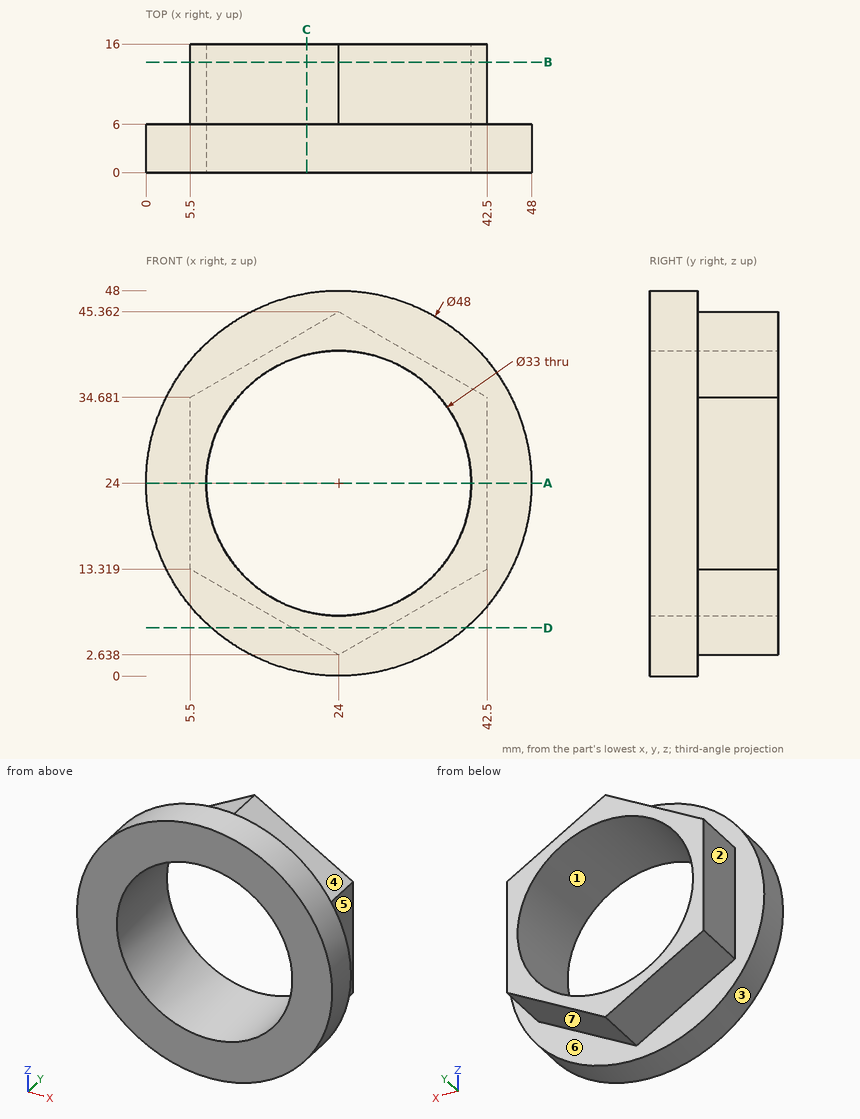
Geometry check sheet. Reference: drawing and pictorial views, mm from the part's lowest x, y, z. A direction names the side the tool comes from. Give positions to 0.01 mm unless a question says otherwise; leave off trailing zeros. Order: outer loops, then holes, each group sorted by start corner. A loop starts at its lowest first (then second) coordinate and runs counter-clockwise, first axis right, second up. Notation, with made-up numbers: M 51,0.5 L 67,0.5 A5 cw 67,4.5 Z; hole C 26,18 d1. An arc over 180 degrees is marked long. Answer in a Markdown table with one row per item. Add a question column.
Q1. Release check for a two-part mould opening along X. For the marked faces 1, 2 and 3 record: released by +X, released by -X, zero draft, split by the parting line, or undercut.
Q2. Sectioned sample at A-A, the plane z = 24. Record the boundary of the cut face in (x, y).
Q3. Thickness scan on L1, parallel to X at y = 10.5, z = 24; L2, parallel to X at y = 3.75, z = 23.5; L3, parallel to Z at x = 24, y = 5. Record the ranges inside material, lowest first.
Q4. Sectioned sample at B-B, the plane y = 13.75. Record the boundary of the cut face in (x, z).
Q5. Sectioned sample at D-D, the plane z = 6. Record the boundary of the cut face in (x, y), and give its area (3 significant figures).
Q6. Access from +Z, -Z, +X, -X, +Y, -Y to the whole of each face (thin tool, end or side, straight path). Record for the marked faces 4, 5, 6 and 7.
Q7. Gauge pin test, flat ends, axial feed: pin 1 Ø4 at (x, z) = (8, 6) entering from +Y; pin 2 Ø6 at (x, z) = (18, 33) entering from -Y; pin 3 Ø6 at (x, y) = (20, 12) entering from -Z; pin 4 Ø1 at (y, z) = (10, 6.5) entering from +X. Record the tip position at first contact, or that the pin passes through.
Q8. Sectioned sample at C-C, the plane x = 20. Record the boundary of the cut face in (y, z).
Verdict:
| question | item | result |
|---|---|---|
| 1 | face 1 | undercut |
| 1 | face 2 | released by -X |
| 1 | face 3 | split by the parting line |
| 2 | outline | M 0,0 L 7.5,0 L 7.5,16 L 5.5,16 L 5.5,6 L 0,6 Z; M 40.5,0 L 48,0 L 48,6 L 42.5,6 L 42.5,16 L 40.5,16 Z |
| 3 | L1 | 5.5 to 7.5, 40.5 to 42.5 |
| 3 | L2 | 0.01 to 7.51, 40.49 to 47.99 |
| 3 | L3 | 0 to 7.5, 40.5 to 48 |
| 4 | outline | M 5.5,13.32 L 24,2.64 L 42.5,13.32 L 42.5,34.68 L 24,45.36 L 5.5,34.68 Z; hole C 24,24 d33 |
| 5 | outline | M 8.13,0 L 39.87,0 L 39.87,6 L 29.82,6 L 29.82,16 L 18.18,16 L 18.18,6 L 8.13,6 Z |
| 5 | area | 307 mm² |
| 6 | face 4 | +Z, +X, +Y |
| 6 | face 5 | +Z, -Z, +X, +Y |
| 6 | face 6 | +Y |
| 6 | face 7 | -Z, +X, +Y |
| 7 | pin 1 | y = 6 |
| 7 | pin 2 | through |
| 7 | pin 3 | z = 3.22 |
| 7 | pin 4 | x = 31.56 |
| 8 | outline | M 0,0.34 L 6,0.34 L 6,4.95 L 16,4.95 L 16,7.99 L 0,7.99 Z; M 0,40.01 L 16,40.01 L 16,43.05 L 6,43.05 L 6,47.66 L 0,47.66 Z |
